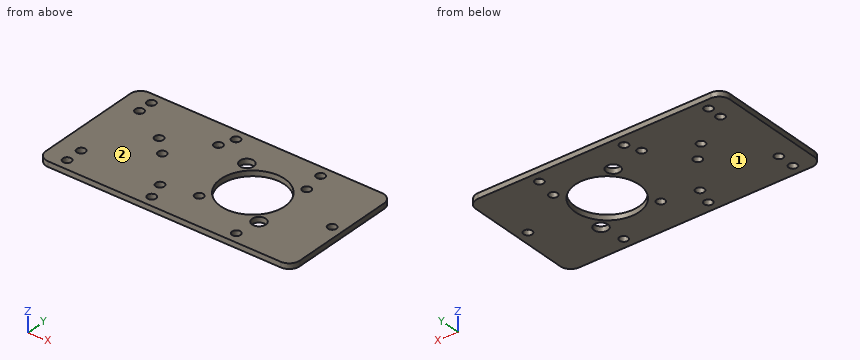
```python
from build123d import *

# Parameters (mm, degrees)
SKETCH1_R           = 2.5527
SKETCH1_R_2         = 4.1275
SKETCH1_R_3         = 19.177
BOSS_EXTRUDE1_DEPTH = 3.175


with BuildPart() as part:
    # Sketch1 → Boss-Extrude1 (new body)
    with BuildSketch(Plane.XY):
        with BuildLine():
            Line((-24.769458796, 9.859734844), (-24.769458796, 73.359734844))
            ThreePointArc((-24.769458796, 73.359734844), (-22.909586857, 77.849862904), (-18.419458796, 79.709734844))
            Line((-18.419458796, 79.709734844), (121.280541204, 79.709734844))
            ThreePointArc((121.280541204, 79.709734844), (125.770669264, 77.849862904), (127.630541204, 73.359734844))
            Line((127.630541204, 73.359734844), (127.630541204, 9.859734844))
            ThreePointArc((127.630541204, 9.859734844), (125.770669264, 5.369606783), (121.280541204, 3.509734844))
            Line((121.280541204, 3.509734844), (-18.419458796, 3.509734844))
            ThreePointArc((-18.419458796, 3.509734844), (-22.909586857, 5.369606783), (-24.769458796, 9.859734844))
        make_face()
        with Locations((89.530541204, 9.859734844)):
            Circle(SKETCH1_R, mode=Mode.SUBTRACT)
        with Locations((89.530541204, 73.359734844)):
            Circle(SKETCH1_R, mode=Mode.SUBTRACT)
        with Locations((-12.069458796, 73.359734844)):
            Circle(SKETCH1_R, mode=Mode.SUBTRACT)
        with Locations((-12.069458796, 64.427395008)):
            Circle(SKETCH1_R, mode=Mode.SUBTRACT)
        with Locations((38.730541204, 73.359734844)):
            Circle(SKETCH1_R, mode=Mode.SUBTRACT)
        with Locations((35.301541204, 64.427395008)):
            Circle(SKETCH1_R, mode=Mode.SUBTRACT)
        with Locations((9.774192889, 51.727395008)):
            Circle(SKETCH1_R, mode=Mode.SUBTRACT)
        with Locations((19.299192889, 42.202395008)):
            Circle(SKETCH1_R, mode=Mode.SUBTRACT)
        with Locations((-12.069458796, 20.433674276)):
            Circle(SKETCH1_R, mode=Mode.SUBTRACT)
        with Locations((35.301541204, 20.433674276)):
            Circle(SKETCH1_R, mode=Mode.SUBTRACT)
        with Locations((38.730541204, 9.859734844)):
            Circle(SKETCH1_R, mode=Mode.SUBTRACT)
        with Locations((55.695028962, 24.33315969)):
            Circle(SKETCH1_R, mode=Mode.SUBTRACT)
        with Locations((55.695028962, 60.254184174)):
            Circle(SKETCH1_R_2, mode=Mode.SUBTRACT)
        with Locations((91.616053446, 60.254184174)):
            Circle(SKETCH1_R, mode=Mode.SUBTRACT)
        with Locations((91.616053446, 24.33315969)):
            Circle(SKETCH1_R_2, mode=Mode.SUBTRACT)
        with Locations((73.655541204, 42.202395008)):
            Circle(SKETCH1_R_3, mode=Mode.SUBTRACT)
        with Locations((-12.069458796, 9.859734844)):
            Circle(SKETCH1_R, mode=Mode.SUBTRACT)
        with Locations((121.280541204, 42.202395008)):
            Circle(SKETCH1_R, mode=Mode.SUBTRACT)
    extrude(amount=BOSS_EXTRUDE1_DEPTH)


solid = part.part
```
Can you work these out from the model? Positions are in its coordinate system, mm. Face numbers are marked on the shaded views. Give positions to 0.01 mm unless a question says otherwise; leave off trailing zeros. Loops run counter-clockwise (first coordinate to the right, second up) from the corner with the lowest first, then second, coordinate; pieces in that order, holes last. Notation, with made-up numbers: M 68,-26.75 L 94,-26.75 A10 ccw 94,-10.75 Z; hole C 42,69.25 d5. An arc over 180 degrees is marked long. Use CSV: the item, a comma, the result in double quotes. Start each with the question number.
1. If I drill on L1, parallel to X at y = 9, z = 2.5; L2, parallel to X at y = 22, z = 2.9; L3, parallel to X at y = 28, z = 2, over which ranges is the centre line in solid material (lowest first)?
2. Imagine slicing it at B-B, the plane z = 1.9. Count the separate pieces of the cut face and the enclosed holes in it, plus the area to 3 significant figures.
3. Imagine slicing it at A-A, the plane y = 32. Write out the boundary of the cut face in (x, z) (3 decimals), plus the area to 3 significant figures.
4. If we mould it in two halves opening along Z, with no side actions, what happens to the marked faces 1 and 2? For each: released by +Z, released by -Z, zero draft, split by the parting line, or undercut.
5. Imagine slicing it at C-C, the plane x = 10. Write out the boundary of the cut face in (y, z) (3 decimals), plus the area to 3 significant figures.
Response values:
1,L1,"-24.71 to -14.47, -9.67 to 36.33, 41.13 to 87.13, 91.93 to 127.57"
1,L2,"-24.77 to -14.09, -10.05 to 33.29, 37.32 to 54.66, 56.73 to 88.21, 95.02 to 127.63"
1,L3,"-24.77 to 60.77, 86.54 to 89.72, 93.51 to 127.63"
2,separate pieces,"1"
2,enclosed holes,"18"
2,area,"10,000 mm^2"
3,outline,"M -24.769,0 L 57.418,0 L 57.418,3.175 L -24.769,3.175 Z; M 89.893,0 L 127.631,0 L 127.631,3.175 L 89.893,3.175 Z"
3,area,"381 mm^2"
4,face 1,"released by -Z"
4,face 2,"released by +Z"
5,outline,"M 3.51,0 L 49.185,0 L 49.185,3.175 L 3.51,3.175 Z; M 54.27,0 L 79.71,0 L 79.71,3.175 L 54.27,3.175 Z"
5,area,"226 mm^2"
